Source: three-view drawing plus pictorial views. Frame: mm from the lowest corner of the part. A direction names the side the tool comes from. Coordinates: 2 decimals unless noted, no trailing zeros. Order: outer loops, then holes, each group sorted by start corner. A loop starts at its lowest first (then second) coordinate and runs counter-clockwise, first axis right, second up. Notation, with made-up numbers: (21, 27.25) - (29, 27.25) arc R36 ccw to (29, 66.25) - close; hole circle Ø1 at (-13, 59.5). An arc over 180 degrees is marked (long way). Use a Markdown table: item, result. Add a question column.
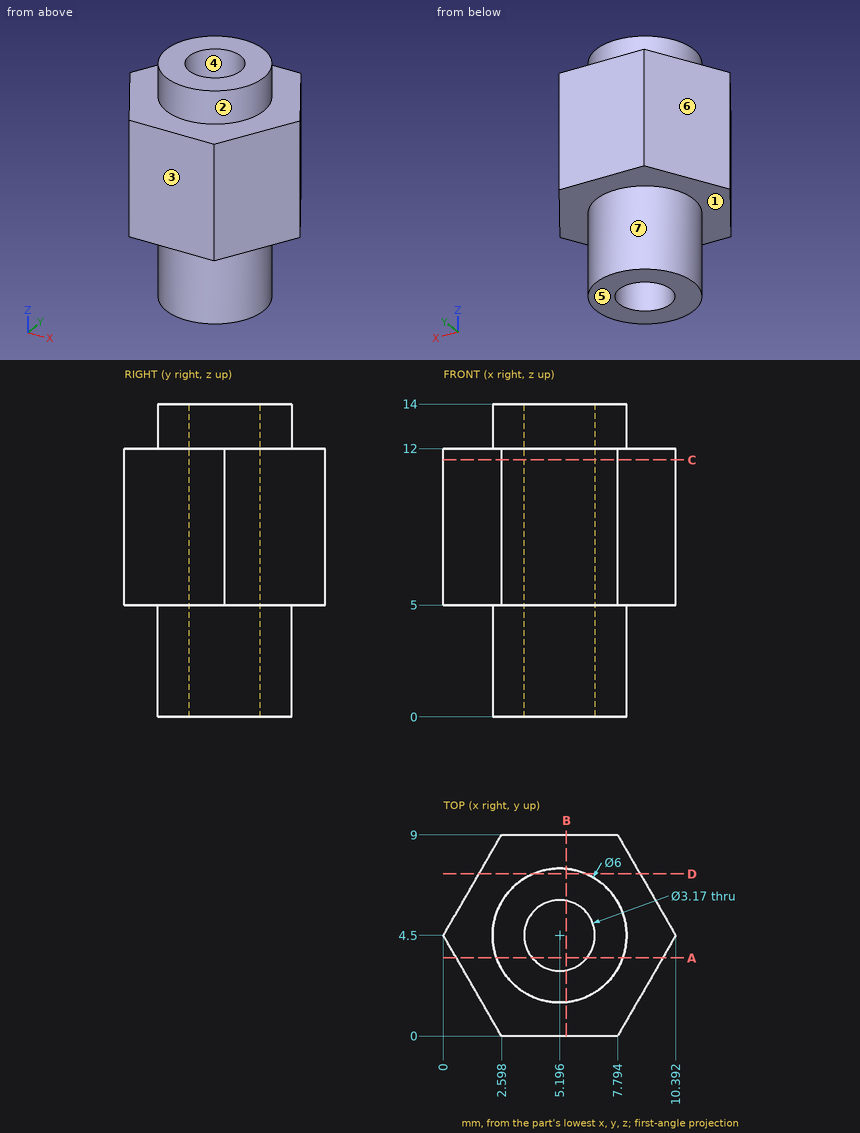
1) Set-up query: the marked faces 1, 2 and 3. Return all of +Z, -Z, +X, -X, +Y, -Y with unobstructed straight access to the full face (end or side cutting, diameter ignored); none if empty.
2) Section C-C (z = 11.5). Return loops of the section in (x, y) (1 decimal).
3) Section D-D (y = 7.25). Return loops of the section in (x, z) (1 decimal), then the cut area to 3 significant figures.
4) Pin query (flat end, axial travel): pin 1 (2 mm diameter, centred on y = 7, z = 11, fed in from -X) (1 decimal). Return the tip coordinate at first contact, or that it passes through.
5) Section A-A (y = 3.5). Return loops of the section in (x, z) (1 decimal).
6) Ray query, line 1 along X through (y, z) = (3.5, 12.5) (1 decimal); line 2 along Y through (x, z) = (5.25, 1.25); line 3 along Z through (x, y) = (1.25, 6). Return the intervals inside material, ascending.
7) Draft query along Y for the marked faces 4, 5, 6 and 7. Return one class per face: pulls with the +Y half, pulls with the -Y half, needs draft (parallel to the pull), parting line crosses it, or undercut.
8) Section B-B (x = 5.5). Return loops of the section in (y, z) (1 decimal).
Values follow:
| question | item | result |
|---|---|---|
| 1 | face 1 | -Z |
| 1 | face 2 | +Z |
| 1 | face 3 | +Z, -Z, +X, -X, -Y |
| 2 | outline | (0, 4.5) - (2.6, 0) - (7.8, 0) - (10.4, 4.5) - (7.8, 9) - (2.6, 9) - close; hole circle Ø3.2 at (5.2, 4.5) |
| 3 | outline | (1.6, 5) - (4, 5) - (4, 0) - (6.4, 0) - (6.4, 5) - (8.8, 5) - (8.8, 12) - (6.4, 12) - (6.4, 14) - (4, 14) - (4, 12) - (1.6, 12) - close |
| 3 | area | 67.3 mm² |
| 4 | pin 1 | stops at x = 0.9 |
| 5 | outline | (0.6, 5) - (2.4, 5) - (2.4, 0) - (4, 0) - (4, 14) - (2.4, 14) - (2.4, 12) - (0.6, 12) - close; (6.4, 0) - (8, 0) - (8, 5) - (9.8, 5) - (9.8, 12) - (8, 12) - (8, 14) - (6.4, 14) - close |
| 6 | line 1 | x = 2.4 to 4, 6.4 to 8 |
| 6 | line 2 | y = 1.5 to 2.92, 6.08 to 7.5 |
| 6 | line 3 | z = 5 to 12 |
| 7 | face 4 | undercut |
| 7 | face 5 | needs draft |
| 7 | face 6 | pulls with the +Y half |
| 7 | face 7 | parting line crosses it |
| 8 | outline | (0, 5) - (1.5, 5) - (1.5, 0) - (2.9, 0) - (2.9, 14) - (1.5, 14) - (1.5, 12) - (0, 12) - close; (6.1, 0) - (7.5, 0) - (7.5, 5) - (9, 5) - (9, 12) - (7.5, 12) - (7.5, 14) - (6.1, 14) - close |
